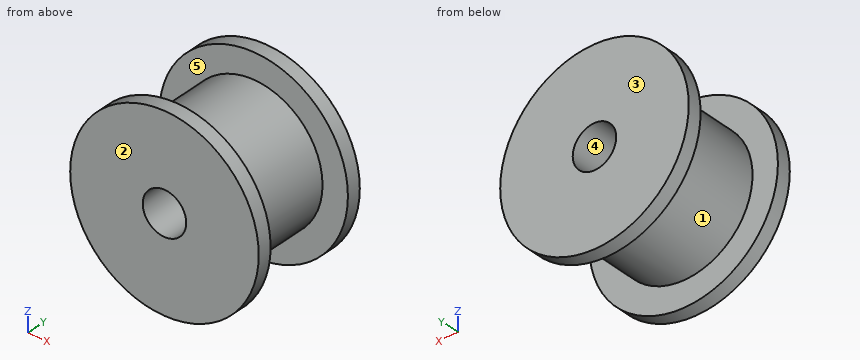
Autodesk Inventor part; units mm, degrees
ref_plane "YZ Plane" through (0, 0, 0) normal (1, 0, 0) x (0, 1, 0)
ref_plane "XZ Plane" through (0, 0, 0) normal (0, 1, 0) x (-1, 0, 0)
ref_plane "XY Plane" through (0, 0, 0) normal (0, 0, 1) x (1, 0, 0)
sketch "Sketch1" plane through (0, 0, 0) normal (0, 1, 0) x (-1, 0, 0)
  circle A0 centre (0, 0) radius 6.5
  dimension "d0" = 13
extrude "Extrusion1" add sketch "Sketch1" along normal blind 1
sketch "Sketch2" plane through (0, 1, 0) normal (0, 1, 0) x (1, 0, 0)
  circle A0 centre (0, 0) radius 4.75
  dimension "d3" = 9.5
extrude "Extrusion2" add sketch "Sketch2" along normal blind 6.5
sketch "Sketch3" plane through (0, 7.5, 0) normal (0, 1, 0) x (1, 0, 0)
  circle A0 centre (0, 0) radius 4.75
  circle A1 centre (0, 0) radius 6.5
extrude "Extrusion3" add sketch "Sketch3" along normal blind 1 contours A0 | A1
sketch "Sketch4" plane through (0, 8.5, 0) normal (0, 1, 0) x (1, 0, 0)
  circle A0 centre (0, 0) radius 1.5
  dimension "d8" = 3
extrude "Extrusion4" cut sketch "Sketch4" against normal blind 10
properties part number "2GT_wheel1"
For this review, take the finished solid that the model builds, in its own axes (mm). Face numbers are marked on the shaded views. A direction names the side the tool comes from. Coordinates: 2 decimals unless noted, no trailing zeros. Loops run counter-clockwise (first coordinate to the right, second up) from the corner with the lowest first, then second, coordinate; pieces in that order, holes last.
1. Add section B-B, the plane z = 0. Give the boundary of the cut face in (x, y), then the cut area to 4 significant figures.
2. Mouldability with a two-part tool opening along Y and no side actions: class the marked faces 3, 4 and 5 as +Y half, -Y half, draft (parallel to the pull), parting line (faces both ways), or undercut.
3. For line 1 (Y direction, x = 5.25, z = -2.25); line 2 (Z direction, x = 0, y = 5.75), list the stretches that pass through material, from the lowest coordinate up.
4. Add section A-A, the plane x = 0. Give the boundary of the cut face in (y, z), then the cut area to 4 significant figures.
5. Add section D-D, the plane z = 1.75. Give the boundary of the cut face in (x, y).
6. Add section C-C, the plane y = 0.75. Give the boundary of the cut face in (x, z), then the cut area to 3 significant figures.
7. For the marked faces 1 and 2, list the 3-axis set-ups (+Z, -Z, +X, -X, +Y, -Y) from which the entire face can be reached by the end or side of a thin tool; tool diameter is ignored.
8. Insertion check: P1, Ø2, axis at x = 3, y = 6, coming from the -Z side; P2, Ø2, axis at y = 4, z = -1, coming from the -X side; P3, Ø5, axis at y = 7, z = -4, coming from the -X side; P4, Ø2.5, axis at x = 0, z = 0, coming from the +Y side. Each pin has a flat end and moves straight along its axis. Give the tip position at first contact, or say it passes through.
Result:
1. outline: (-6.5, 0) - (-1.5, 0) - (-1.5, 8.5) - (-6.5, 8.5) - (-6.5, 7.5) - (-4.75, 7.5) - (-4.75, 1) - (-6.5, 1) - close; (1.5, 0) - (6.5, 0) - (6.5, 1) - (4.75, 1) - (4.75, 7.5) - (6.5, 7.5) - (6.5, 8.5) - (1.5, 8.5) - close
1. area: 62.25 mm2
2. face 3: +Y half
2. face 4: draft
2. face 5: undercut
3. line 1: y = 0 to 1, 7.5 to 8.5
3. line 2: z = -4.75 to -1.5, 1.5 to 4.75
4. outline: (0, -6.5) - (1, -6.5) - (1, -4.75) - (7.5, -4.75) - (7.5, -6.5) - (8.5, -6.5) - (8.5, -1.5) - (0, -1.5) - close; (0, 1.5) - (8.5, 1.5) - (8.5, 6.5) - (7.5, 6.5) - (7.5, 4.75) - (1, 4.75) - (1, 6.5) - (0, 6.5) - close
4. area: 62.25 mm2
5. outline: (-6.26, 0) - (6.26, 0) - (6.26, 1) - (4.42, 1) - (4.42, 7.5) - (6.26, 7.5) - (6.26, 8.5) - (-6.26, 8.5) - (-6.26, 7.5) - (-4.42, 7.5) - (-4.42, 1) - (-6.26, 1) - close
6. outline: circle Ø13 at (0, 0); hole circle Ø3 at (0, 0)
6. area: 126 mm2
7. face 1: none
7. face 2: +Z, -Z, +X, -X, -Y
8. P1: stops at z = -4.31
8. P2: stops at x = -4.75
8. P3: stops at x = -6.31
8. P4: passes through
